Check sheet for the modelled part. Datum: model origin and axes. Units: mm. Give positions to 0.01 mm unless a question says otherwise; leave off trailing zeros. Order: outer loops, then holes, each group sorted by start corner. A loop starts at its lowest first (then second) coordinate and runs counter-clockwise, first axis right, second up.
from build123d import *

# Parameters (mm, degrees)
CROQUIS1_R               = 1.6
SALIENTE_EXTRUIR1_DEPTH  = 2
REDONDEO1_R              = 3
CROQUIS3_W               = 19
CROQUIS3_H               = 38
SORTIDA_CABLE_LLIT_DEPTH = 3
REDONDEO3_R              = 3
CROQUIS4_W               = 6
CROQUIS4_H               = 6
FORAT_TERMISTOR_DEPTH    = 3
REDONDEO4_R              = 1


with BuildPart() as part:
    # Croquis1 → Saliente-Extruir1 (new body)
    with BuildSketch(Plane(origin=(0, 2, 0), x_dir=(1, 0, 0), z_dir=(0, 1, 0))):
        Polygon((0, 198), (0, 108), (18, 108), (18, 90), (0, 90), (0, 0), (267, 0), (267, 18), (285, 18), (285, 180), (267, 180), (267, 198), align=None)
        with Locations((142.5, 193.5)):
            Circle(CROQUIS1_R, mode=Mode.SUBTRACT)
        with Locations((4.5, 193.5)):
            Circle(CROQUIS1_R, mode=Mode.SUBTRACT)
        with Locations((280.5, 22.5)):
            Circle(CROQUIS1_R, mode=Mode.SUBTRACT)
        with Locations((280.5, 175.5)):
            Circle(CROQUIS1_R, mode=Mode.SUBTRACT)
        with Locations((280.5, 99)):
            Circle(CROQUIS1_R, mode=Mode.SUBTRACT)
        with Locations((142.5, 4.5)):
            Circle(CROQUIS1_R, mode=Mode.SUBTRACT)
        with Locations((4.5, 4.5)):
            Circle(CROQUIS1_R, mode=Mode.SUBTRACT)
        with Locations((142.5, 99)):
            Circle(CROQUIS1_R, mode=Mode.SUBTRACT)
        with Locations((22.5, 99)):
            Circle(CROQUIS1_R, mode=Mode.SUBTRACT)
    extrude(amount=-SALIENTE_EXTRUIR1_DEPTH)

    # Redondeo1
    redondeo1_edges = [part.edges().sort_by_distance(p)[0] for p in [
        (267, 1, -198),
        (267, 1, -180),
        (285, 1, -180),
        (285, 1, -18),
        (267, 1, -18),
        (267, 1, 0),
        (0, 1, 0),
        (0, 1, -90),
        (18, 1, -90),
        (18, 1, -108),
        (0, 1, -108),
        (0, 1, -198),
    ]]
    fillet(redondeo1_edges, radius=REDONDEO1_R)

    # Croquis3 → Sortida cable llit (cut, through all)
    with BuildSketch(Plane(origin=(0, 2, 0), x_dir=(1, 0, 0), z_dir=(0, 1, 0))):
        with Locations((275.5, 138)):
            Rectangle(CROQUIS3_W, CROQUIS3_H)
    extrude(amount=-SORTIDA_CABLE_LLIT_DEPTH, mode=Mode.SUBTRACT)

    # Redondeo3
    redondeo3_edges = [part.edges().sort_by_distance(p)[0] for p in [
        (285, 1, -157),
        (285, 1, -119),
        (266, 1, -119),
        (266, 1, -157),
    ]]
    fillet(redondeo3_edges, radius=REDONDEO3_R)

    # Croquis4 → Forat termistor (cut, through all)
    with BuildSketch(Plane.XZ):
        with Locations((136.5, -93)):
            Rectangle(CROQUIS4_W, CROQUIS4_H)
        with Locations((136.5, -105)):
            Rectangle(CROQUIS4_W, CROQUIS4_H)
    extrude(amount=-FORAT_TERMISTOR_DEPTH, mode=Mode.SUBTRACT)

    # Redondeo4
    redondeo4_edges = [part.edges().sort_by_distance(p)[0] for p in [
        (133.5, 1, -96),
        (133.5, 1, -90),
        (139.5, 1, -90),
        (139.5, 1, -96),
        (139.5, 1, -108),
        (133.5, 1, -108),
        (133.5, 1, -102),
        (139.5, 1, -102),
    ]]
    fillet(redondeo4_edges, radius=REDONDEO4_R)


solid = part.part
1) Section check B-B, the plane y = 0.5. State how many separate pieces and enclosed holes the cut face has, then the cut area to 3 significant figures.
Recorded:
separate pieces: 1
enclosed holes: 11
area: 54,600 mm2
2) Section check A-A, the plane z = -146.5. Record the cut outline in (x, y).
Recorded:
outline: (0, 0) - (266, 0) - (266, 2) - (0, 2) - close
3) Depth check by flat-ended pin: pin 1 Ø1.9 at (x, z) = (142.5, -4.5) entering from +Y; pin 2 Ø1 at (x, y) = (277, 1) entering from +Z. Enter the tip coordinate at first touch or a pass-through.
Recorded:
pin 1: passes through
pin 2: stops at z = -18
4) Material ranges on L1, parallel to Z at x = 4.5, y = 1.2; L2, parallel to Z at x = 142.5, y = 1.5; L3, parallel to X at y = 1.35, z = -99, recorded low to high.
Recorded:
L1: z = -198 to -195.1, -191.9 to -108, -90 to -6.1, -2.9 to 0
L2: z = -198 to -195.1, -191.9 to -100.6, -97.4 to -6.1, -2.9 to 0
L3: x = 18 to 20.9, 24.1 to 140.9, 144.1 to 278.9, 282.1 to 285
